Could you check a few things on this model? Use its own coordinates, in mm. A direction names the side the tool comes from. Give positions to 0.01 mm unless a question says otherwise; leave off trailing zeros. Loops run counter-clockwise (first coordinate to the right, second up) from the corner with the lowest first, then second, coordinate; pieces in that order, holes last. Notation, with made-up numbers: (-5.75, -16) -> (31.25, -16) arc R26 cw to (31.25, 9) -> close; hole circle Ø5 at (-18.75, 64.25). An arc over 180 degrees is marked (long way). Put each result on its own line as item: value.
```python
from build123d import *

# Parameters (mm, degrees)
BOSS_EXTRU_1_DEPTH      = 800
ENL_V_MAT_EXTRU_1_DEPTH = 30
ENL_V_MAT_EXTRU_2_DEPTH = 30
ENL_V_MAT_EXTRU_4_DEPTH = 300
CONG_1_R                = 2


with BuildPart() as part:
    # Esquisse1 → Boss.-Extru.1 (new body)
    with BuildSketch(Plane(origin=(0, 0, 0), x_dir=(0, 0, -1), z_dir=(1, 0, 0))):
        Polygon((0, 0), (230, 0), (230, -55), (227, -55), (227, -3), (3, -3), (3, -55), (0, -55), align=None)
    extrude(amount=BOSS_EXTRU_1_DEPTH)

    # Esquisse2 → Enlèv. mat.-Extru.1 (cut)
    with BuildSketch(Plane(origin=(0, 0, 0), x_dir=(1, 0, 0), z_dir=(0, 1, 0))):
        with BuildLine():
            Line((443.5, 190.5), (543.5, 190.5))
            ThreePointArc((543.5, 190.5), (547.75, 186.25), (543.5, 182))
            Line((543.5, 182), (443.5, 182))
            ThreePointArc((443.5, 182), (439.25, 186.25), (443.5, 190.5))
        make_face()
        with BuildLine():
            Line((640, 190.5), (740, 190.5))
            ThreePointArc((740, 190.5), (744.25, 186.25), (740, 182))
            Line((740, 182), (640, 182))
            ThreePointArc((640, 182), (635.75, 186.25), (640, 190.5))
        make_face()
        with BuildLine():
            Line((443.5, 88.5), (543.5, 88.5))
            ThreePointArc((543.5, 88.5), (547.75, 84.25), (543.5, 80))
            Line((543.5, 80), (443.5, 80))
            ThreePointArc((443.5, 80), (439.25, 84.25), (443.5, 88.5))
        make_face()
        with BuildLine():
            Line((640, 88.5), (740, 88.5))
            ThreePointArc((740, 88.5), (744.25, 84.25), (740, 80))
            Line((740, 80), (640, 80))
            ThreePointArc((640, 80), (635.75, 84.25), (640, 88.5))
        make_face()
    extrude(amount=-ENL_V_MAT_EXTRU_1_DEPTH, mode=Mode.SUBTRACT)

    # Esquisse3 → Enlèv. mat.-Extru.2 (cut)
    with BuildSketch(Plane(origin=(0, 0, 0), x_dir=(1, 0, 0), z_dir=(0, 1, 0))):
        with BuildLine():
            Line((70, 217.1), (70, 167.1))
            ThreePointArc((70, 167.1), (65, 162.1), (60, 167.1))
            Line((60, 167.1), (60, 217.1))
            ThreePointArc((60, 217.1), (65, 222.1), (70, 217.1))
        make_face()
        with BuildLine():
            Line((270, 217.1), (270, 167.1))
            ThreePointArc((270, 167.1), (265, 162.1), (260, 167.1))
            Line((260, 167.1), (260, 217.1))
            ThreePointArc((260, 217.1), (265, 222.1), (270, 217.1))
        make_face()
        with BuildLine():
            Line((270, 85.2), (270, 35.2))
            ThreePointArc((270, 35.2), (265, 30.2), (260, 35.2))
            Line((260, 35.2), (260, 85.2))
            ThreePointArc((260, 85.2), (265, 90.2), (270, 85.2))
        make_face()
        with BuildLine():
            Line((60, 35.2), (60, 85.2))
            ThreePointArc((60, 85.2), (65, 90.2), (70, 85.2))
            Line((70, 85.2), (70, 35.2))
            ThreePointArc((70, 35.2), (65, 30.2), (60, 35.2))
        make_face()
    extrude(amount=-ENL_V_MAT_EXTRU_2_DEPTH, mode=Mode.SUBTRACT)

    # Esquisse6 → Enlèv. mat.-Extru.4 (cut)
    with BuildSketch(Plane.XY):
        with BuildLine():
            Line((595, -55), (605, -55))
            Line((605, -55), (610, -55))
            Line((610, -55), (605, -45))
            Line((605, -45), (605, -35))
            ThreePointArc((605, -35), (600, -30), (595, -35))
            Line((595, -35), (595, -45))
            Line((595, -45), (590, -55))
            Line((590, -55), (595, -55))
        make_face()
        with BuildLine():
            Line((110, -45), (105, -55))
            Line((105, -55), (110, -55))
            Line((110, -55), (120, -55))
            Line((120, -55), (125, -55))
            Line((125, -55), (120, -45))
            Line((120, -45), (120, -35))
            ThreePointArc((120, -35), (115, -30), (110, -35))
            Line((110, -35), (110, -45))
        make_face()
    extrude(amount=-ENL_V_MAT_EXTRU_4_DEPTH, mode=Mode.SUBTRACT)

    # Congé1
    cong_1_edges = [part.edges().sort_by_distance(p)[0] for p in [
        (400, 0, 0),
        (400, 0, -230),
    ]]
    fillet(cong_1_edges, radius=CONG_1_R)


solid = part.part
```
1. Thinking about a two-plate mould opening in Z: for faces 1 (the face through (394, -29, -3)), 2 (the face through (394, -29, 0)), 3 (the face through (394, 0, -113)), which applies, pulls with the +Z half, pulls with the -Z half, needs draft (parallel to the pull), parting line crosses it, or undercut?
Recorded:
face 1: undercut
face 2: pulls with the +Z half
face 3: needs draft
2. If we section it at C-C (x = 696): List the corners of the cut face in (y, z) for me.
Recorded:
outline: (-55, -230) -> (-2, -230) arc R2 ccw to (0, -228) -> (0, -190.5) -> (-3, -190.5) -> (-3, -227) -> (-55, -227) -> close; (-55, -3) -> (-3, -3) -> (-3, -80) -> (0, -80) -> (0, -2) arc R2 ccw to (-2, 0) -> (-55, 0) -> close; (-3, -182) -> (0, -182) -> (0, -88.5) -> (-3, -88.5) -> close
3. I'm going to push flat-ended pins straight in: pin 1 (0.9 mm diameter, centred on x = 475, y = -1, fed in from +Z); pin 2 (6 mm diameter, centred on x = 661.5, z = -30.5, fed in from -Y). Where does each tip first touch, or does it pass through?
Recorded:
pin 1: stops at z = -0.08
pin 2: stops at y = -3
4. I need wall thicknesses on line 1 (Z direction, x = 736, y = -38.5); line 2 (Y direction, x = 504, z = -113.5). Which ranges of each line are inside material? Lowest first, please.
Recorded:
line 1: z = -230 to -227, -3 to 0
line 2: y = -3 to 0
5. For faces 4 (the face through (394, -3, -117)), 5 (the face through (0, -1, -116)), which set-ups out of +Z, -Z, +X, -X, +Y, -Y let a thin tool reach every point of the face, with its end or its side?
Recorded:
face 4: +X, -X, -Y
face 5: +Z, -Z, -X, +Y, -Y
6. If we section it at D-D (x = 583): List the corners of the cut face in (y, z) for me, then the cut area to 3 significant figures.
Recorded:
outline: (-55, -230) -> (-2, -230) arc R2 ccw to (0, -228) -> (0, -2) arc R2 ccw to (-2, 0) -> (-55, 0) -> (-55, -3) -> (-3, -3) -> (-3, -227) -> (-55, -227) -> close
area: 1,000 mm^2
7. If we section it at B-B (y = -17): List the corners of the cut face in (x, z) for me, then the cut area to 3 significant figures.
Recorded:
outline: (0, -230) -> (800, -230) -> (800, -227) -> (0, -227) -> close; (0, -3) -> (800, -3) -> (800, 0) -> (0, 0) -> close
area: 4,800 mm^2
8. If we section it at A-A (z = -48): List the corners of the cut face in (x, y) for me, then the cut area to 3 significant figures.
Recorded:
outline: (0, -3) -> (60, -3) -> (60, 0) -> (0, 0) -> close; (70, -3) -> (260, -3) -> (260, 0) -> (70, 0) -> close; (270, -3) -> (800, -3) -> (800, 0) -> (270, 0) -> close
area: 2,340 mm^2
